Check sheet for the modelled part. Datum: model origin and axes. Units: mm. A direction names the side the tool comes from. Coordinates: 2 decimals unless noted, no trailing zeros. Order: outer loops, then holes, each group sorted by start corner. A loop starts at its lowest first (then second) coordinate and runs counter-clockwise, first axis right, second up. Notation, with made-up numbers: (-22.75, 5) -> (-16.75, 5) arc R25 cw to (-16.75, 34) -> close; hole circle Ø9 at (-3, 44.25). An arc over 180 degrees is marked (long way). Put each result on its own line as item: value. Start each with the question number.
```python
from build123d import *

# Parameters (mm, degrees)
F0_R     = 17.8054
F1_DEPTH = 19
F2_R     = 5
F3_DEPTH = 3
F4_R     = 1
F5_DEPTH = 16.6116


with BuildPart() as f1:
    # F0 (on Front) → F1 (new body, symmetric)
    with BuildSketch(Plane.XZ):
        Circle(F0_R)
    extrude(amount=F1_DEPTH, both=True)

    # F2 (on face) → F3 (join)
    with BuildSketch(Plane.XZ.offset(19)):
        Circle(F2_R)
    extrude(amount=F3_DEPTH)

    # F4 (on face) → F5 (join)
    with BuildSketch(Plane.XZ.offset(22)):
        Circle(F4_R)
    extrude(amount=F5_DEPTH)


solid = f1.part
```
1) Sectioned sample at B-B (x = 0). Record the boundary of the cut face in (y, z).
2) Sectioned sample at A-A (z = 0). Record the boundary of the cut face in (x, y), plus the area to 3 significant figures.
3) Sectioned sample at C-C (y = -12.5). Record the boundary of the cut face in (x, z), plus the area to 3 significant figures.
4) Sectioned sample at D-D (y = -21). Record the boundary of the cut face in (x, z), plus the area to 3 significant figures.
5) Scan lines: line 1 along Y through (x, z) = (4, -8); line 2 along X through (y, z) = (-2, 7). Record each from-to range of solid material in increasing order. Write a range as [from, to].
6) Gauge pin test, flat ends, axial feed: pin 1 (4 mm diameter, centred on x = 7, y = -20, fed in from +Z); pin 2 (1.5 mm diameter, centred on x = -1.5, y = 8.5, fed in from -Z); pin 3 (5 mm diameter, centred on x = 7.5, y = 11, fed in from +Z); pin 4 (18 mm diameter, centred on x = -0.5, z = 4, fed in from -Y). Record the tip position at first contact, or that the pin passes through.
7) Access from +Z, -Z, +X, -X, +Y, -Y to the whole of each face (thin tool, end or side, straight path). Record for faces 1 (the cylindrical face through (-1.08, -20.48, -4.88)), 2 (the flat face through (0, -38.612, 0)).
Entries:
1. outline: (-38.61, -1) -> (-22, -1) -> (-22, -5) -> (-19, -5) -> (-19, -17.81) -> (19, -17.81) -> (19, 17.81) -> (-19, 17.81) -> (-19, 5) -> (-22, 5) -> (-22, 1) -> (-38.61, 1) -> close
2. outline: (-17.81, -19) -> (-5, -19) -> (-5, -22) -> (-1, -22) -> (-1, -38.61) -> (1, -38.61) -> (1, -22) -> (5, -22) -> (5, -19) -> (17.81, -19) -> (17.81, 19) -> (-17.81, 19) -> close
2. area: 1,420 mm2
3. outline: circle Ø35.61 at (0, 0)
3. area: 996 mm2
4. outline: circle Ø10 at (0, 0)
4. area: 78.5 mm2
5. line 1: y = [-19, 19]
5. line 2: x = [-16.37, 16.37]
6. pin 1: stops at z = 17.01
6. pin 2: stops at z = -17.79
6. pin 3: stops at z = 17.09
6. pin 4: stops at y = -38.61
7. face 1: -Y
7. face 2: +Z, -Z, +X, -X, -Y
